Work out the finished part from the listing and answer in its coordinate system (mm). A direction names the side the tool comes from. Coordinates: 2 decimals unless noted, no trailing zeros. Write each loop counter-clockwise with the first axis right and the second up, starting at its lowest first coordinate (ties: lowest second). Pieces come first, ordered by that corner, then holes. Notation, with made-up numbers: (-21, 85.5) - (12, 85.5) arc R36 ccw to (12, 121.5) - close; hole circle Ø10 at (33, 78.5). An arc over 180 degrees is marked (long way). One line per item, written item: value.
```python
from build123d import *

# Parameters (mm, degrees)
F0_W     = 450
F0_H     = 900
F1_DEPTH = 225
F2_W     = 50
F2_H     = 50
F2_H_2   = 400
F2_W_2   = 330
F3_DEPTH = 450.001
F4_W     = 380
F4_H     = 400
F5_DEPTH = 450.001
F6_W     = 380
F6_H     = 277.7692569069
F6_H_2   = 50
F7_DEPTH = 134.1753041809


# Not quite as in the source:
# - a feature names something its author has since deleted; it is built from what else it names


with BuildPart() as f1:
    # F0 (on Front) → F1 (new body, symmetric)
    with BuildSketch(Plane.XZ):
        with Locations((0, 450)):
            Rectangle(F0_W, F0_H)
    extrude(amount=F1_DEPTH, both=True)

    # F2 (on face) → F3 (cut, through all)
    with BuildSketch(Plane.YZ.offset(225)):
        Polygon((-225, 450), (140, 450), (190, 900), (-225, 900), align=None)
        Polygon((175, 450), (225, 450), (225, 900), align=None)
        with Locations((200, 425)):
            Rectangle(F2_W, F2_H)
        with Locations((200, 200)):
            Rectangle(F2_W, F2_H_2)
        with Locations((-25, 200)):
            Rectangle(F2_W_2, F2_H_2)
    extrude(amount=-F3_DEPTH, mode=Mode.SUBTRACT)

    # F4 (on face) → F5 (cut, through all)
    with BuildSketch(Plane.XZ.offset(225)):
        with Locations((0, 200)):
            Rectangle(F4_W, F4_H)
    extrude(amount=-F5_DEPTH, mode=Mode.SUBTRACT)

    # F6 (on face) → F7 (cut, through all)
    with BuildSketch(Plane(origin=(0, 88.9024390244, -9.8780487805), x_dir=(1, 0, 0), z_dir=(0, -0.9938837347, 0.1104315261))):
        with Locations((0, 601.592722707)):
            Rectangle(F6_W, F6_H)
        with Locations((0, 815.4773511605)):
            Rectangle(F6_W, F6_H_2)
    extrude(amount=-F7_DEPTH, mode=Mode.SUBTRACT)


solid = f1.part
```
Item 1: Section D-D, the plane y = 100.5 is taken. Determine the outline of the cut face in (x, z), then the cut area to 3 significant figures.
Evaluation:
outline: (-225, 400) - (225, 400) - (225, 450) - (-225, 450) - close
area: 22,500 mm2
Item 2: Section B-B, the plane x = 123.5 is taken. Determine the outline of the cut face in (y, z).
Evaluation:
outline: (-225, 400) - (175, 400) - (175, 446.11) - (140, 450) - (-225, 450) - close; (170.67, 726.07) - (205.25, 722.23) - (210.77, 771.92) - (176.2, 775.76) - close; (181.72, 825.46) - (216.29, 821.62) - (225, 900) - (190, 900) - close
Item 3: Section A-A, the plane z = 213 is taken. Determine the outline of the cut face in (x, y), then the cut area to 3 significant figures.
Evaluation:
outline: (-225, -225) - (-190, -225) - (-190, -190) - (-225, -190) - close; (-225, 140) - (-190, 140) - (-190, 175) - (-225, 175) - close; (190, -225) - (225, -225) - (225, -190) - (190, -190) - close; (190, 140) - (225, 140) - (225, 175) - (190, 175) - close
area: 4,900 mm2
Item 4: Consider probe 1 along Y at (x, z) = (200, 94); probe 2 along Z at (x, y) = (29.5, -2); probe 3 along Y at (x, z) = (-124, 767). Determine where each line is inside the solid, lowest interval first.
Evaluation:
probe 1: y = -225 to -190, 140 to 175
probe 2: z = 400 to 450
probe 3: y = 175.22 to 210.22
Item 5: Section C-C, the plane z = 797.5 is taken. Determine the outline of the cut face in (x, y), then the cut area to 3 significant figures.
Evaluation:
outline: (-225, 178.61) - (-190, 178.61) - (-190, 213.61) - (-225, 213.61) - close; (190, 178.61) - (225, 178.61) - (225, 213.61) - (190, 213.61) - close
area: 2,450 mm2
Item 6: Given pin 1 (17.5 mm diameter, centred on x = -206, z = 180.5, fed in from +Y); pin 2 (3 mm diameter, centred on x = -55.5, y = 1, fed in from +Z), each flat-ended and moving along its own axis, determine where each tip first touches the part or whether it passes through.
Evaluation:
pin 1: stops at y = 175
pin 2: stops at z = 450
Item 7: Which of the six approach directions +Z, -Z, +X, -X, +Y, -Y give full straight-line access (tool end or side, diameter ignored) to faces 1 (the face through (3, -45, 450)), 2 (the face through (207, 157, 0)), 3 (the face through (1, 175, 409)), 4 (the face through (225, 49, 415)), 5 (the face through (-207, -190, 197))?
Evaluation:
face 1: +Z, +X, -X, -Y
face 2: -Z, +X, -X, +Y, -Y
face 3: -Z, +X, -X, +Y
face 4: +Z, -Z, +X, +Y, -Y
face 5: -Z, +X, -X
Item 8: Determine the mould class of faces 6 (the face through (190, -208, 197)), 7 (the face through (3, -28, 400)), 8 (the face through (-1, -225, 409)), 9 (the face through (-225, 49, 415)) for opening direction X: +X half, -X half, draft (parallel to the pull), parting line (faces both ways), or undercut.
Evaluation:
face 6: undercut
face 7: undercut
face 8: draft
face 9: -X half
